Geometry check sheet. Reference: the model listing, model coordinates, mm. A direction names the side the tool comes from. Round coordinates to 2 decimals unless told otherwise and drop trailing zeros. Loops run counter-clockwise (first coordinate to the right, second up) from the corner with the lowest first, then second, coordinate; pieces in that order, holes last. Notation, with made-up numbers: (5.25, 41.5) -> (32.25, 41.5) arc R29 ccw to (32.25, 64.5) -> close; hole circle Ø10 at (63.25, -13.75). An arc over 180 degrees is marked (long way). Use one line per item in the form item = value.
from build123d import *

# Parameters (mm, degrees)
BOSS_EXTRUDE1_DEPTH      = 6.686777
BOSS_EXTRUDE1_DEPTH_BACK = 0.0001
SKETCH1_W                = 11.6
SKETCH1_H                = 30.55
SKETCH2_W                = 4.6
SKETCH2_H                = 21
BOSS_EXTRUDE3_DEPTH      = 10
FILLET1_R                = 3
SKETCH3_W                = 4.6
SKETCH3_H                = 4.4
SKETCH3_H_2              = 2.05
BOSS_EXTRUDE4_DEPTH      = 4.113123252
SKETCH4_W                = 3.1
SKETCH4_H                = 3.586876748
CUT_EXTRUDE1_DEPTH       = 87.944077783
SKETCH5_R                = 1.6
CUT_EXTRUDE2_DEPTH       = 87.944077783
SKETCH6_R                = 1
CUT_EXTRUDE3_DEPTH       = 91.600623245
FILLET2_R                = 1
FILLET3_R                = 3
FILLET4_R                = 2
CHAMFER1_SIZE            = 2.5
FILLET5_R                = 0.8


with BuildPart() as part:
    # Sketch1 → Boss-Extrude1 (new, two sides: drawn at the far end of the back side and taken through both)
    with BuildSketch(Plane(origin=(0, 0, 0), x_dir=(1, 0, 0), z_dir=(0, 1, 0)).offset(-BOSS_EXTRUDE1_DEPTH_BACK)):
        with Locations((22.195659191, -69.260579157)):
            Rectangle(SKETCH1_W, SKETCH1_H)
    extrude(amount=BOSS_EXTRUDE1_DEPTH + BOSS_EXTRUDE1_DEPTH_BACK)

    # Sketch2 → Boss-Extrude3 (add)
    with BuildSketch(Plane(origin=(0, 6.686776748, 0), x_dir=(1, 0, 0), z_dir=(0, 1, 0))):
        with Locations((25.695659191, -74.035579157)):
            Rectangle(SKETCH2_W, SKETCH2_H)
    extrude(amount=BOSS_EXTRUDE3_DEPTH)

    # Fillet1
    fillet1_edges = [part.edges().sort_by_distance(p)[0] for p in [
        (23.395659191, 16.686776748, 74.035579157),
    ]]
    fillet(fillet1_edges, radius=FILLET1_R)

    # Sketch3 → Boss-Extrude4 (add)
    with BuildSketch(Plane(origin=(0, 6.686776748, 0), x_dir=(1, 0, 0), z_dir=(0, 1, 0))):
        with Locations((25.695659191, -56.185579157)):
            Rectangle(SKETCH3_W, SKETCH3_H)
        with Locations((25.695659191, -62.510579157)):
            Rectangle(SKETCH3_W, SKETCH3_H_2)
    extrude(amount=BOSS_EXTRUDE4_DEPTH)

    # Sketch4 → Cut-Extrude1 (cut, through all)
    with BuildSketch(Plane(origin=(27.995659191, 0, 0), x_dir=(0, 0, -1), z_dir=(1, 0, 0))):
        with Locations((-59.935579157, 4.893338374)):
            Rectangle(SKETCH4_W, SKETCH4_H)
    extrude(amount=-CUT_EXTRUDE1_DEPTH, mode=Mode.SUBTRACT)

    # Sketch5 → Cut-Extrude2 (cut, through all)
    with BuildSketch(Plane(origin=(27.995659191, 0, 0), x_dir=(0, 0, -1), z_dir=(1, 0, 0))):
        with Locations((-68.535579157, 11.686776748)):
            Circle(SKETCH5_R)
        with Locations((-79.535579157, 11.686776748)):
            Circle(SKETCH5_R)
    extrude(amount=-CUT_EXTRUDE2_DEPTH, mode=Mode.SUBTRACT)

    # Sketch6 → Cut-Extrude3 (cut, through all)
    with BuildSketch(Plane.XZ.offset(0.0001)):
        with Locations(Location((21.895659191, 59.935579157, 0), (0, 0, 270))):
            Circle(SKETCH6_R)
        with Locations(Location((21.895659191, 71.935579157, 0), (0, 0, 270))):
            Circle(SKETCH6_R)
    extrude(amount=-CUT_EXTRUDE3_DEPTH, mode=Mode.SUBTRACT)

    # Fillet2
    fillet2_edges = [part.edges().sort_by_distance(p)[0] for p in [
        (25.695659191, 10.7999, 58.385579157),
        (25.695659191, 10.7999, 53.985579157),
        (25.695659191, 10.7999, 61.485579157),
        (25.695659191, 10.7999, 63.535579157),
    ]]
    fillet(fillet2_edges, radius=FILLET2_R)

    # Fillet3
    fillet3_edges = [part.edges().sort_by_distance(p)[0] for p in [
        (16.395659191, 6.686777, 73.010579157),
        (16.395659191, 6.686777, 56.185579157),
        (23.395659191, 6.686776748, 56.185579157),
    ]]
    fillet(fillet3_edges, radius=FILLET3_R)

    # Fillet4
    fillet4_edges = [part.edges().sort_by_distance(p)[0] for p in [
        (16.395659191, 3.0999, 59.935579157),
    ]]
    fillet(fillet4_edges, radius=FILLET4_R)

    # Chamfer1
    chamfer1_edges = [part.edges().sort_by_distance(p)[0] for p in [
        (27.995659191, 11.686776748, 70.135579157),
        (27.995659191, 11.686776748, 81.135579157),
    ]]
    chamfer(chamfer1_edges, length=CHAMFER1_SIZE)

    # Fillet5
    fillet5_edges = [part.edges().sort_by_distance(p)[0] for p in [
        (27.995659191, 10.7999, 56.185579157),
        (27.995659191, 6.4499, 58.385579157),
        (27.995659191, 6.4499, 61.485579157),
        (27.995659191, 10.7999, 62.510579157),
        (27.995659191, 10.507006781, 58.092685938),
        (27.995659191, 10.507006781, 61.778472375),
        (27.995659191, 10.507006781, 54.278472375),
        (27.995659191, 11.092793218, 63.242685938),
        (27.995659191, 14.243338374, 63.535579157),
        (27.995659191, 16.686776748, 74.035579157),
        (27.995659191, 8.343338374, 84.535579157),
        (27.995659191, 4.8999, 53.985579157),
        (27.995659191, 3.0999, 59.935579157),
    ]]
    fillet(fillet5_edges, radius=FILLET5_R)


solid = part.part
1. Section check C-C (z = 74). Record the boundary of the cut face in (x, y).
Return value:
outline = (16.4, 0) -> (28, 0) -> (28, 15.89) arc R0.8 ccw to (27.2, 16.69) -> (26.4, 16.69) arc R3 ccw to (23.4, 13.69) -> (23.4, 6.69) -> (19.4, 6.69) arc R3 ccw to (16.4, 3.69) -> close
2. Material ranges on line 1 along Z through (x, y) = (25.5, 4.75); line 2 along Z through (x, y) = (25.75, 10.5); line 3 along Y through (x, z) = (19.25, 61), recorded low to high.
Return value:
line_1 = 53.99 to 58.39, 61.49 to 84.54
line_2 = 54.27 to 58.1, 61.77 to 67.11, 69.96 to 78.11, 80.96 to 84.54
line_3 = 0 to 3.1
3. Mould release check, pull along Z, two halves, no side actions. Record for faces 5 (the cylindrical face through (21.513, 1.528, 59.012)), 6 (the flat face through (23, 6, 84.536)), 7 (the flat face through (21, 6.687, 73)), 8 (the cylindrical face through (25.3, 10.5, 58.1)): released by +Z, released by -Z, zero draft, split by the parting line, or undercut.
Return value:
face_5 = undercut
face_6 = released by +Z
face_7 = zero draft
face_8 = undercut
4. Tool access check on faces 1 (the cylindrical face through (17, 2.53, 59.96)), 2 (the flat face through (27.996, 6, 69)), 3 (the flat face through (25, 14, 63.536)), 4 (the flat face through (23, 3.1, 59)). Record the directions out of +Z, -Z, +X, -X, +Y, -Y that give a thin tool (end or side, any length) a straight path to the whole face; none if there is none.
Return value:
face_1 = -X, +Y
face_2 = +Z, -Z, +X, +Y, -Y
face_3 = -Z, +X, -X, +Y
face_4 = +X, -X, +Y
5. Section check D-D (x = 25). Record the boundary of the cut face in (y, z).
Return value:
outline = (0, 53.99) -> (9.8, 53.99) arc R1 ccw to (10.8, 54.99) -> (10.8, 57.39) arc R1 ccw to (9.8, 58.39) -> (3.1, 58.39) -> (3.1, 61.49) -> (9.8, 61.49) arc R1 ccw to (10.8, 62.49) -> (10.8, 62.54) arc R1 cw to (11.8, 63.54) -> (16.34, 63.54) -> (16.34, 84.54) -> (0, 84.54) -> close; hole circle Ø3.2 at (11.69, 68.54); hole circle Ø3.2 at (11.69, 79.54)
6. Gauge pin test, flat ends, axial feed: pin 1 (10 mm diameter, centred on y = 15, z = 77.5, fed in from -X); pin 2 (1.9 mm diameter, centred on x = 25, y = 15, fed in from -Z); pin 3 (0.7 mm diameter, centred on x = 26, z = 56, fed in from +Y). Record the tip position at first contact, or that the pin passes through.
Return value:
pin_1 = 23.4
pin_2 = 63.54
pin_3 = 10.8
7. Section check A-A (x = 19.75). Record the boundary of the cut face in (y, z), then the cut area to 3 significant figures.
Return value:
outline = (0, 53.99) -> (6.69, 53.99) -> (6.69, 58.39) -> (3.1, 58.39) -> (3.1, 61.49) -> (6.69, 61.49) -> (6.69, 84.54) -> (0, 84.54) -> close
area = 193 mm2
8. Section check B-B (y = 2). Record the boundary of the cut face in (x, z).
Return value:
outline = (16.4, 53.99) -> (27.2, 53.99) arc R0.8 ccw to (28, 54.79) -> (28, 83.74) arc R0.8 ccw to (27.2, 84.54) -> (16.4, 84.54) -> (16.4, 61.49) -> (16.61, 61.49) -> (16.61, 58.39) -> (16.4, 58.39) -> close; hole circle Ø2 at (21.9, 59.94); hole circle Ø2 at (21.9, 71.94)
